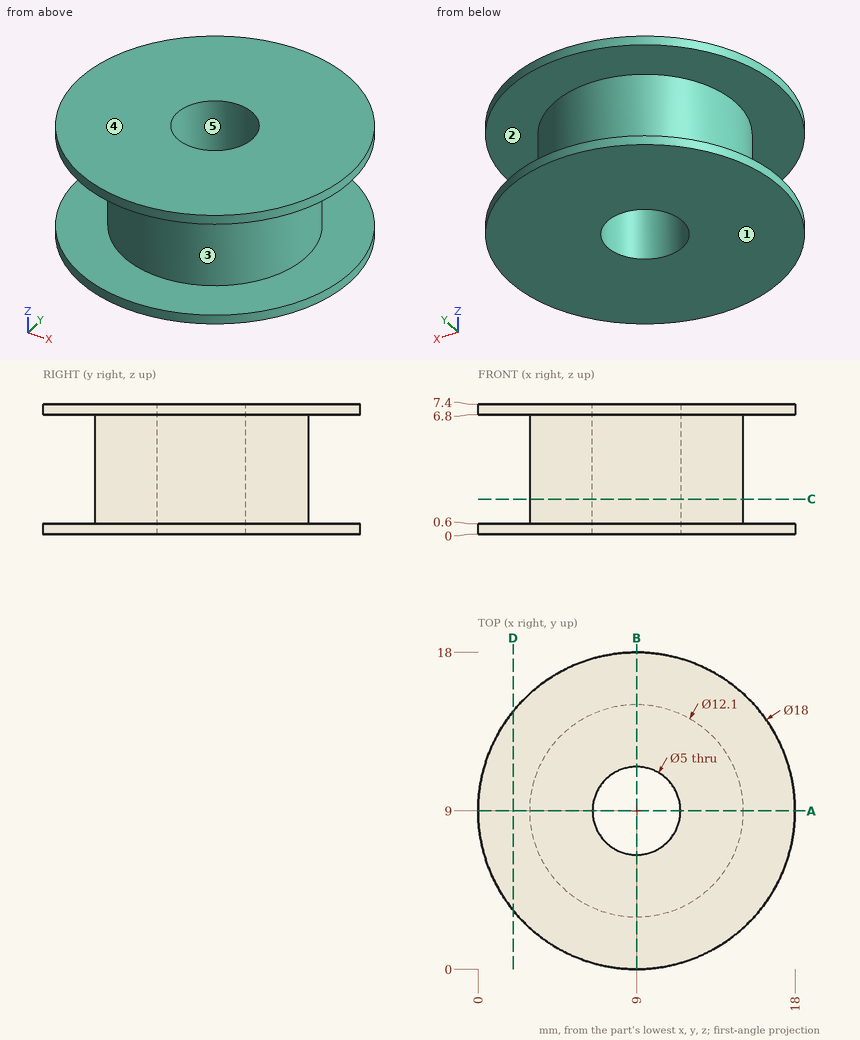
Job drawing, mm, ordinate dimensions from the low corner. One solid piece. A direction names the side the tool comes from. Give positions to 0.01 mm unless a question says otherwise; leave off trailing zeros. Loops run counter-clockwise (first coordinate to the right, second up) from the corner with the lowest first, then second, coordinate; pieces in that order, holes last. Notation, with made-up numbers: M 56,3.25 L 64,3.25 A23 ccw 64,36.25 Z; hole C 50.5,80 d11. An arc over 180 degrees is marked long. Use one line per item in the form item = value.
Item 1: Two-plate mould, pull along Y, no slides. Class the marked faces 3, 4 and 5: released by +Y, released by -Y, zero draft, split by the parting line, or undercut.
Filled in:
face_3 = split by the parting line
face_4 = zero draft
face_5 = undercut
Item 2: Slice it at D-D on x = 2. List the corners of the cut face in (y, z), and give its area (3 significant figures).
Filled in:
outline = M 3.34,0 L 14.66,0 L 14.66,0.6 L 3.34,0.6 Z; M 3.34,6.8 L 14.66,6.8 L 14.66,7.4 L 3.34,7.4 Z
area = 13.6 mm^2
Item 3: Flat gauge pin, fed straight in: pin 1 Ø4.5 at (x, y) = (9, 9) entering from +Z. Where does the tip first touch, or does it go through?
Filled in:
pin_1 = through
Item 4: Which spindle directions (+Z, -Z, +X, -X, +Y, -Y) get a long thin tool onto all of the face, cutting with end or side? Do the marked faces 1 and 2. Say none if no direction does.
Filled in:
face_1 = -Z, +X, -X, +Y, -Y
face_2 = none
Item 5: Slice it at C-C on z = 2. List the corners of the cut face in (x, y).
Filled in:
outline = C 9,9 d12.1; hole C 9,9 d5
Item 6: Slice it at A-A on y = 9. List the corners of the cut face in (x, z).
Filled in:
outline = M 0,0 L 6.5,0 L 6.5,7.4 L 0,7.4 L 0,6.8 L 2.95,6.8 L 2.95,0.6 L 0,0.6 Z; M 11.5,0 L 18,0 L 18,0.6 L 15.05,0.6 L 15.05,6.8 L 18,6.8 L 18,7.4 L 11.5,7.4 Z
Item 7: Drill centre lines: L1, parallel to Z at x = 1, y = 8.25; L2, parallel to Y at x = 9, z = 5.25; L3, parallel to Y at x = 9.75, z = 2.5. Where is each one in solid material? Low to high.
Filled in:
L1 = 0 to 0.6, 6.8 to 7.4
L2 = 2.95 to 6.5, 11.5 to 15.05
L3 = 3 to 6.62, 11.38 to 15
